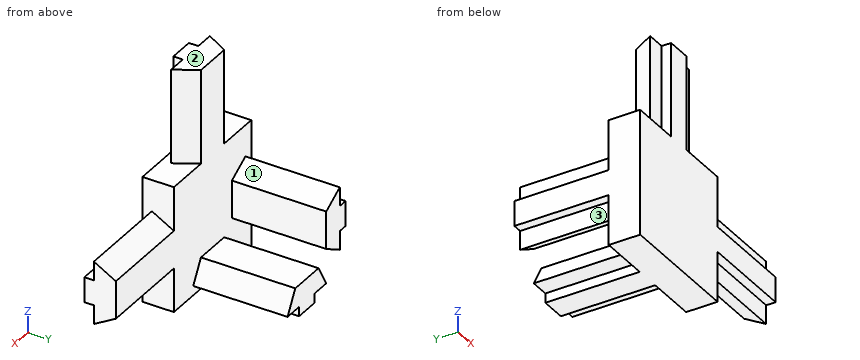
```python
from build123d import *

# Parameters (mm, degrees)
SKETCH1_W           = 20
SKETCH1_H           = 20
BOSS_EXTRUDE1_DEPTH = 2.5
BOSS_EXTRUDE2_DEPTH = 15
CIRPATTERN1_COUNT   = 2
CIRPATTERN1_ANGLE   = 90
BOSS_EXTRUDE3_DEPTH = 15
CIRPATTERN2_COUNT   = 2
CIRPATTERN2_ANGLE   = 90


with BuildPart() as part:
    # Sketch1 → Boss-Extrude1 (new, symmetric)
    with BuildSketch(Plane(origin=(0, 0, 0), x_dir=(1, 0, 0), z_dir=(0, 1, 0))):
        Rectangle(SKETCH1_W, SKETCH1_H)
    extrude(amount=BOSS_EXTRUDE1_DEPTH, both=True)

    # Sketch2 → Boss-Extrude2 (add)
    with BuildSketch(Plane(origin=(0, 2.5, 0), x_dir=(1, 0, 0), z_dir=(0, 1, 0))):
        Polygon((-2, 10), (2, 10), (2, 8.5), (5, 8.5), (3, 5), (-3, 5), (-5, 8.5), (-2, 8.5), align=None)
    boss_extrude2 = extrude(amount=BOSS_EXTRUDE2_DEPTH)

    # CirPattern1: Boss-Extrude2 ×2 about axis
    cirpattern1_axis = Axis((0, 0, 0), (0, 1, 0))
    for i in range(1, CIRPATTERN1_COUNT):
        add(boss_extrude2.rotate(cirpattern1_axis, i * CIRPATTERN1_ANGLE / (CIRPATTERN1_COUNT - 1)))

    # Sketch3 → Boss-Extrude3 (add)
    with BuildSketch(Plane(origin=(10, 0, 0), x_dir=(0, 0, -1), z_dir=(1, 0, 0))):
        Polygon((-3, 2.5), (3, 2.5), (5, -1), (2, -1), (2, -2.5), (-2, -2.5), (-2, -1), (-5, -1), align=None)
    boss_extrude3 = extrude(amount=BOSS_EXTRUDE3_DEPTH)

    # CirPattern2: Boss-Extrude3 ×2 about axis
    cirpattern2_axis = Axis((0, 0, 0), (0, -1, 0))
    for i in range(1, CIRPATTERN2_COUNT):
        add(boss_extrude3.rotate(cirpattern2_axis, i * CIRPATTERN2_ANGLE / (CIRPATTERN2_COUNT - 1)))


solid = part.part
```
Could you check a few things on this model? Use its own coordinates, in mm. Face numbers are marked on the shaded views. A direction names the side the tool comes from. Coordinates: 2 decimals unless noted, no trailing zeros. Write each loop counter-clockwise with the first axis right and the second up, starting at its lowest first coordinate (ties: lowest second). Pieces come first, ordered by that corner, then holes. Notation, with made-up numbers: (9.25, 29.25) -> (53.25, 29.25) arc R26 ccw to (53.25, 54.25) -> close; hole circle Ø7 at (44.25, -38.75). An arc over 180 degrees is marked (long way). Return JSON: item names as keys, results as strings.
(1) Which directions (+Z, -Z, +X, -X, +Y, -Y) give clear straight access to the entire face, cutting with the end or side of a thin tool? Please do the marked faces 1, 2 and 3.
Numbers:
{"face 1": "+Z, +X, +Y", "face 2": "+Z, +X, -X, +Y, -Y", "face 3": "-Z, -X, +Y"}
(2) Imagine slicing it at D-D, the plane z = -4. Please give me the cut outline in (x, y), then the cut area to 4 significant figures.
Numbers:
{"outline": "(-10, -2.5) -> (10, -2.5) -> (10, -1) -> (25, -1) -> (25, 0.75) -> (10, 0.75) -> (10, 2.5) -> (-6.75, 2.5) -> (-6.75, 17.5) -> (-8.5, 17.5) -> (-8.5, 2.5) -> (-10, 2.5) -> close", "area": "152.5 mm2"}
(3) I need wall thicknesses on L1, parallel to Y at x = 0, z = 0; L2, parallel to Z at x = -1, y = 12; L3, parallel to Z at x = -5.5, y = 1.5. Which ranges of each line are inside material? Lowest first, please.
Numbers:
{"L1": "y = -2.5 to 2.5", "L2": "z = -10 to -5", "L3": "z = -10 to 10"}
(4) Imagine slicing it at A-A, the plane y = 12.25. Please give me the cut outline in (x, z), then the cut area to 3 significant figures.
Numbers:
{"outline": "(-10, -2) -> (-8.5, -2) -> (-8.5, -5) -> (-5, -3) -> (-5, 3) -> (-8.5, 5) -> (-8.5, 2) -> (-10, 2) -> close; (-5, -8.5) -> (-2, -8.5) -> (-2, -10) -> (2, -10) -> (2, -8.5) -> (5, -8.5) -> (3, -5) -> (-3, -5) -> close", "area": "68.0 mm2"}
(5) Imagine slicing it at C-C, the plane z = 15. Please give me the cut outline in (x, y), then the cut area to 3 significant figures.
Numbers:
{"outline": "(-5, -1) -> (-2, -1) -> (-2, -2.5) -> (2, -2.5) -> (2, -1) -> (5, -1) -> (3, 2.5) -> (-3, 2.5) -> close", "area": "34.0 mm2"}
(6) Imagine slicing it at B-B, the plane x = 14. Please give me the cut outline in (y, z), then the cut area to 3 significant figures.
Numbers:
{"outline": "(-2.5, -2) -> (-1, -2) -> (-1, -5) -> (2.5, -3) -> (2.5, 3) -> (-1, 5) -> (-1, 2) -> (-2.5, 2) -> close", "area": "34.0 mm2"}
(7) I'm going to push flat-ended pins straight in: pin 1 (2.5 mm diameter, centred on y = 11.5, z = -4, fed in from -X); pin 2 (0.8 mm diameter, centred on y = 9, z = -9.5, fed in from -X); pin 3 (5 mm diameter, centred on x = 6, z = 16.5, fed in from -Y); pin 4 (10 mm diameter, centred on y = 13, z = 12, fed in from +X). Where does each tip first touch, or does it pass through?
Numbers:
{"pin 1": "stops at x = -8.5", "pin 2": "stops at x = -2", "pin 3": "stops at y = -1", "pin 4": "passes through"}
